The drawing under review shows one solid part. Ordinate dimensions are in mm from its lowest x, y, z. A direction names the side the tool comes from. Give positions to 0.01 mm unless a question says otherwise; leave off trailing zeros. Write each loop counter-clockwise with the first axis right and the second up, starting at its lowest first coordinate (ties: lowest second). Pieces come first, ordered by that corner, then holes. Notation, with made-up numbers: (67, -4) -> (117, -4) arc R21 ccw to (117, 31) -> close; hole circle Ø11 at (65.25, 38.25). An arc over 180 degrees is marked (long way). Use CSV: the item, a comma, the result in double quotes.
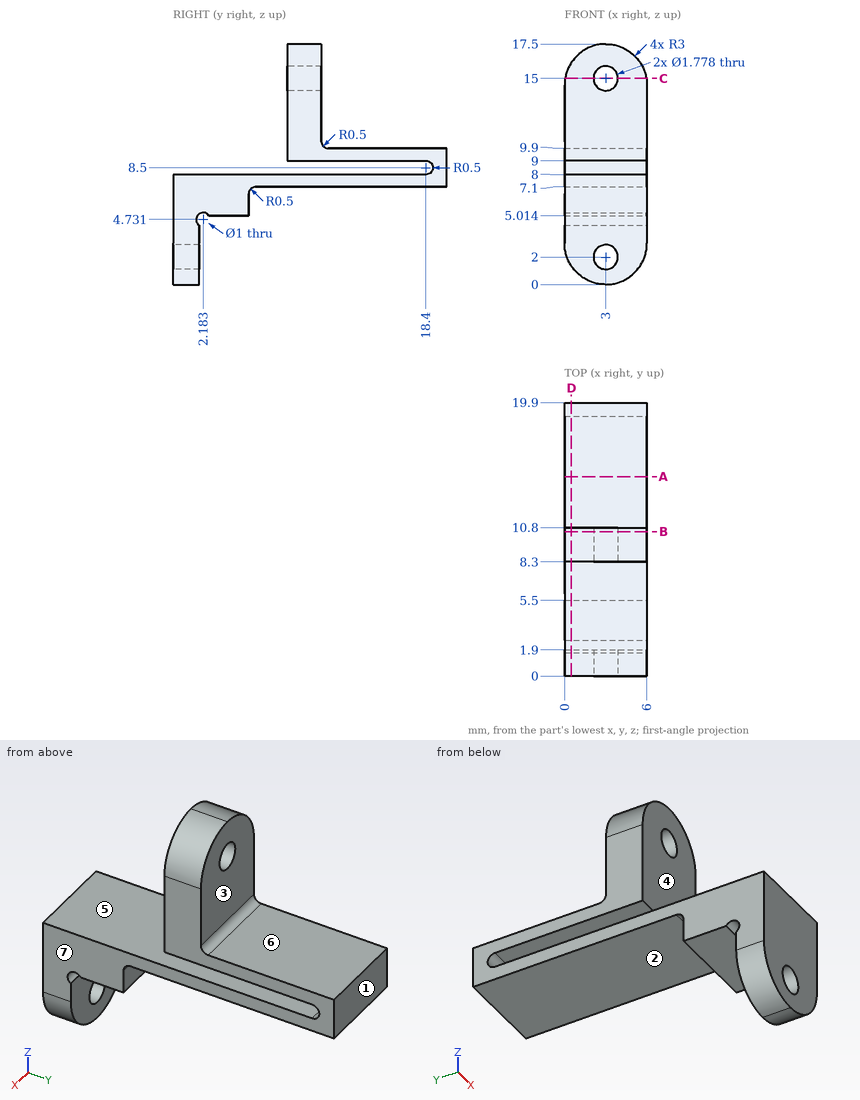
(1) Take a section at C-C (z = 15). Write out the cut boundary in (x, y).
Established:
outline,"(0.04, 8.3) -> (2.11, 8.3) -> (2.11, 10.8) -> (0.04, 10.8) -> close; (3.89, 8.3) -> (5.96, 8.3) -> (5.96, 10.8) -> (3.89, 10.8) -> close"
(2) Tool access review of the marked faces 1, 2, 3 and 4: name each direction out of +Z, -Z, +X, -X, +Y, -Y from which nothing blocks a thin tool from reaching the whole face with its end or side.
Established:
face 1,"+Z, -Z, +X, -X, +Y"
face 2,"-Z, +X, -X, +Y"
face 3,"+Z, +X, -X, +Y"
face 4,"+Z, +X, -X, -Y"
(3) Mouldability with a two-part tool opening along Z and no side actions: class the marked faces 5, 6 and 7 as +Z half, -Z half, draft (parallel to the pull), parting line (faces both ways), or undercut.
Established:
face 5,"undercut"
face 6,"+Z half"
face 7,"draft"
(4) For line 1 along Z through (x, y) = (3, 9.15); line 2 along Z through (x, y) = (3, 0.4); line 3 along Z through (x, y) = (4.75, 11.5), list the stretches that pass through material, from the lowest coordinate up. Write a range as [from, to].
Established:
line 1,"z = [7.1, 8], [9, 14.11], [15.89, 17.5]"
line 2,"z = [0, 1.11], [2.89, 8]"
line 3,"z = [7.1, 8], [9, 9.9]"
(5) Take a section at A-A (y = 14.5). Write out the cut boundary in (x, z), then the cut area to 3 significant figures.
Established:
outline,"(0, 7.1) -> (6, 7.1) -> (6, 8) -> (0, 8) -> close; (0, 9) -> (6, 9) -> (6, 9.9) -> (0, 9.9) -> close"
area,"10.8 mm2"
(6) Take a section at D-D (x = 0.5). Write out the cut boundary in (y, z) (1 decimal).
Established:
outline,"(0, 1.3) -> (1.9, 1.3) -> (1.9, 4.3) arc R0.5 cw (long way) to (2.6, 5) -> (5.5, 5) -> (5.5, 6.6) arc R0.5 cw to (6, 7.1) -> (19.9, 7.1) -> (19.9, 9.9) -> (11.3, 9.9) arc R0.5 cw to (10.8, 10.4) -> (10.8, 16.2) -> (8.3, 16.2) -> (8.3, 9) -> (18.4, 9) arc R0.5 cw to (18.4, 8) -> (0, 8) -> close"
(7) Take a section at B-B (y = 10.5). State how many separate pieces and enclosed holes the cut face has.
Established:
separate pieces,"2"
enclosed holes,"1"
(8) Clearance check with flat-ended pins moving along their axes: pin 1 (1.8 mm diameter, centred on x = 2, y = 13.5, fed in from +Z); pin 2 (3 mm diameter, centred on x = 2.5, y = 10, fed in from -Z); pin 3 (2 mm diameter, centred on y = 15, z = 4.5, fed in from +X); pin 4 (0.5 mm diameter, centred on x = 3, z = 6, fed in from +Y). State where each tip first meets the part, or that it passes through.
Established:
pin 1,"stops at z = 9.9"
pin 2,"stops at z = 7.1"
pin 3,"passes through"
pin 4,"stops at y = 5.5"
